Verification items for the finished model (mm, model axes). Round coordinates to 2 decimals unless told otherwise and drop trailing zeros. Write each loop counter-clockwise with the first axis right and the second up, starting at its lowest first coordinate (ties: lowest second). Pieces come first, ordered by that corner, then holes. Notation, with made-up numbers: M 65.5,13 L 70.5,13 A16 cw 70.5,42 Z; hole C 72,-23 d4. An arc over 180 degrees is marked long. Write each question's results on one line, items separated by ' | '.
from build123d import *

# Parameters (mm, degrees)
SKETCH_1_W          = 54.8
SKETCH_1_H          = 54.8
SKETCH_1_R          = 4.1
SKETCH_1_R_2        = 1.6
EXTRUDE_1_DEPTH     = 4.4
FILLET_1_R          = 6
SKETCH_2_R          = 1.6
CUT_EXTRUDE_1_DEPTH = 10


with BuildPart() as part:
    # 草图1 → 凸台-拉伸1 (new body)
    with BuildSketch(Plane(origin=(0, 0, 0), x_dir=(1, 0, 0), z_dir=(0, 1, 0))):
        Rectangle(SKETCH_1_W, SKETCH_1_H)
        Circle(SKETCH_1_R, mode=Mode.SUBTRACT)
        with Locations((21.4, 21.4)):
            Circle(SKETCH_1_R_2, mode=Mode.SUBTRACT)
        with Locations((21.4, -21.4)):
            Circle(SKETCH_1_R_2, mode=Mode.SUBTRACT)
        with Locations((-21.4, -21.4)):
            Circle(SKETCH_1_R_2, mode=Mode.SUBTRACT)
        with Locations((-21.4, 21.4)):
            Circle(SKETCH_1_R_2, mode=Mode.SUBTRACT)
        Polygon((17.7, -5), (17.7, 5), (17.7, 13), (22.4, 13), (22.4, 5), (22.4, -5), (22.4, -13), (17.7, -13), align=None, mode=Mode.SUBTRACT)
        Polygon((-5, 17.7), (-13, 17.7), (-13, 22.4), (-5, 22.4), (5, 22.4), (13, 22.4), (13, 17.7), (5, 17.7), align=None, mode=Mode.SUBTRACT)
        Polygon((5, -17.7), (13, -17.7), (13, -22.4), (5, -22.4), (-5, -22.4), (-13, -22.4), (-13, -17.7), (-5, -17.7), align=None, mode=Mode.SUBTRACT)
        Polygon((-17.7, 5), (-17.7, -5), (-17.7, -13), (-22.4, -13), (-22.4, -5), (-22.4, 5), (-22.4, 13), (-17.7, 13), align=None, mode=Mode.SUBTRACT)
    extrude(amount=EXTRUDE_1_DEPTH)

    # 圆角1
    fillet_1_edges = [part.edges().sort_by_distance(p)[0] for p in [
        (27.4, 2.2, 27.4),
        (-27.4, 2.2, 27.4),
        (-27.4, 2.2, -27.4),
        (27.4, 2.2, -27.4),
    ]]
    fillet(fillet_1_edges, radius=FILLET_1_R)

    # 草图2 → 切除-拉伸1 (cut)
    with BuildSketch(Plane(origin=(0, 4.4, 0), x_dir=(1, 0, 0), z_dir=(0, 1, 0))):
        with Locations((10.7, 10.7)):
            Circle(SKETCH_2_R)
        with Locations((10.7, -10.7)):
            Circle(SKETCH_2_R)
        with Locations((-10.7, -10.7)):
            Circle(SKETCH_2_R)
        with Locations((-10.7, 10.7)):
            Circle(SKETCH_2_R)
    extrude(amount=-CUT_EXTRUDE_1_DEPTH, mode=Mode.SUBTRACT)


solid = part.part
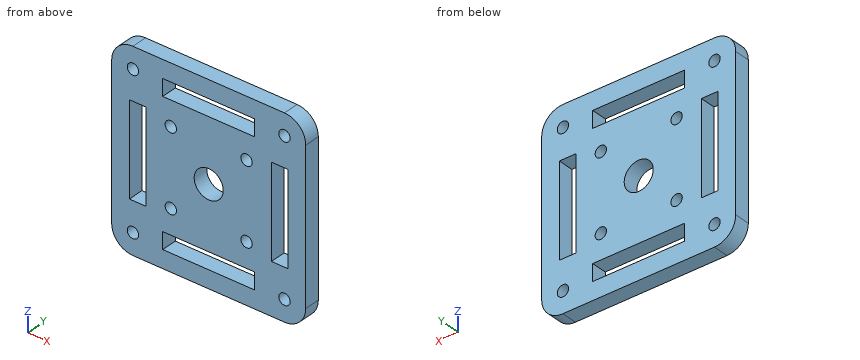
1) Sectioned sample at D-D, the plane x = -10.7. Record the cut outline in (y, z).
Calculated:
outline: M 0,-27.4 L 4.4,-27.4 L 4.4,-22.4 L 0,-22.4 Z; M 0,-17.7 L 4.4,-17.7 L 4.4,-12.3 L 0,-12.3 Z; M 0,-9.1 L 4.4,-9.1 L 4.4,9.1 L 0,9.1 Z; M 0,12.3 L 4.4,12.3 L 4.4,17.7 L 0,17.7 Z; M 0,22.4 L 4.4,22.4 L 4.4,27.4 L 0,27.4 Z
2) Sectioned sample at A-A, the plane x = 0. Record the cut outline in (y, z), and give its area (3 significant figures).
Calculated:
outline: M 0,-27.4 L 4.4,-27.4 L 4.4,-22.4 L 0,-22.4 Z; M 0,-17.7 L 4.4,-17.7 L 4.4,-4.1 L 0,-4.1 Z; M 0,4.1 L 4.4,4.1 L 4.4,17.7 L 0,17.7 Z; M 0,22.4 L 4.4,22.4 L 4.4,27.4 L 0,27.4 Z | area: 164 mm²
3) Sectioned sample at B-B, the plane y = 3.35. Count the separate pieces of the cut face and the enclosed holes in it, and give its area (3 significant figures).
Calculated:
separate pieces: 1 | enclosed holes: 13 | area: 2,370 mm²
4) Depth check by flat-ended pin: P1, Ø12, axis at x = -21.5, z = 0, coming from the +Y side; P2, Ø1.9, axis at x = 10.7, z = 10.7, coming from the +Y side. Enter the tip coordinate at first touch or a pass-through.
Calculated:
P1: stops at y = 4.4 | P2: passes through
5) Material ranges on line 1 (X direction, y = 3.2, z = -21.4); line 2 (X direction, y = 3.1, z = -6); line 3 (X direction, y = 3.4, z = -10.7), recorded low to high. Write a range as [from, to].
Calculated:
line 1: x = [-27.4, -23], [-19.8, -13], [13, 19.8], [23, 27.4] | line 2: x = [-27.4, -22.4], [-17.7, 17.7], [22.4, 27.4] | line 3: x = [-27.4, -22.4], [-17.7, -12.3], [-9.1, 9.1], [12.3, 17.7], [22.4, 27.4]
6) Sectioned sample at C-C, the plane z = 10.7. Record the cut outline in (x, y).
Calculated:
outline: M -27.4,0 L -22.4,0 L -22.4,4.4 L -27.4,4.4 Z; M -17.7,0 L -12.3,0 L -12.3,4.4 L -17.7,4.4 Z; M -9.1,0 L 9.1,0 L 9.1,4.4 L -9.1,4.4 Z; M 12.3,0 L 17.7,0 L 17.7,4.4 L 12.3,4.4 Z; M 22.4,0 L 27.4,0 L 27.4,4.4 L 22.4,4.4 Z
